Part model, mm, in its own coordinate system. Coordinates: 2 decimals unless noted, no trailing zeros. Loops run counter-clockwise (first coordinate to the right, second up) from the corner with the lowest first, then second, coordinate; pieces in that order, holes last. Notation, with made-up numbers: M -32,34 L 20,34 A25 ccw 20,61 Z; hole C 18.5,86 d10. An arc over 180 degrees is marked long. Use a Markdown table: item, result. Add a question column.
1) Band-saw the part on C-C (x = 5). List the corners of the cut face in (y, z).
2) Band-saw the part on A-A (x = 6). List the corners of the cut face in (y, z).
3) Pull direction Z, two halves, no side cores. Call faces 1 (the flat face through (5, 0.463, 1)), 2 (the flat face through (5, 5, 0)), 3 (the flat face through (5, 5, 2.5)): released by +Z, released by -Z, zero draft, split by the parting line, or undercut.
4) Band-saw the part on B-B (y = 1.75). List the corners of the cut face in (x, z).
5) Wall check: probe 1 along X at (y, z) = (8, 1.05); probe 2 along Z at (x, y) = (6.25, 6.25); probe 3 along Y at (x, z) = (2, 1.45). Give the ranges that are in metal, low to high. Write a range as from..to.
from build123d import *

# Parameters (mm, degrees)
CROQUIS1_W              = 9.859
CROQUIS1_H              = 2.5
CROQUIS1_W_2            = 0.636
CROQUIS1_H_2            = 0.636
SALIENTE_EXTRUIR2_DEPTH = 9.6
CHAFL_N2_SIZE           = 0.5
CHAFL_N3_SIZE           = 0.5
CROQUIS2_W              = 1.000954756
CROQUIS2_H              = 0.463176593
CORTAR_EXTRUIR1_DEPTH   = 10.859


with BuildPart() as part:
    # Croquis1 → Saliente-Extruir2 (new body)
    with BuildSketch(Plane(origin=(0, 0, 0), x_dir=(1, 0, 0), z_dir=(0, 1, 0))):
        with Locations((4.9295, -1.25)):
            Rectangle(CROQUIS1_W, CROQUIS1_H)
        with Locations((1.118, -1.25)):
            Rectangle(CROQUIS1_W_2, CROQUIS1_H_2, mode=Mode.SUBTRACT)
        with Locations((3.659, -1.25)):
            Rectangle(CROQUIS1_W_2, CROQUIS1_H_2, mode=Mode.SUBTRACT)
        with Locations((8.741, -1.25)):
            Rectangle(CROQUIS1_W_2, CROQUIS1_H_2, mode=Mode.SUBTRACT)
        with Locations((6.2, -1.25)):
            Rectangle(CROQUIS1_W_2, CROQUIS1_H_2, mode=Mode.SUBTRACT)
    extrude(amount=SALIENTE_EXTRUIR2_DEPTH)

    # Chaflán2
    chafl_n2_edges = [part.edges().sort_by_distance(p)[0] for p in [
        (0.8, 9.6, 1.25),
        (1.118, 9.6, 1.568),
        (1.436, 9.6, 1.25),
        (1.118, 9.6, 0.932),
    ]]
    chamfer(chafl_n2_edges, length=CHAFL_N2_SIZE)

    # Chaflán3
    chafl_n3_edges = [part.edges().sort_by_distance(p)[0] for p in [
        (3.659, 9.6, 0.932),
        (3.341, 9.6, 1.25),
        (3.659, 9.6, 1.568),
        (3.977, 9.6, 1.25),
        (8.741, 9.6, 0.932),
        (8.423, 9.6, 1.25),
        (8.741, 9.6, 1.568),
        (9.059, 9.6, 1.25),
        (6.2, 9.6, 0.932),
        (5.882, 9.6, 1.25),
        (6.2, 9.6, 1.568),
        (6.518, 9.6, 1.25),
    ]]
    chamfer(chafl_n3_edges, length=CHAFL_N3_SIZE)

    # Croquis2 → Cortar-Extruir1 (cut, through all)
    with BuildSketch(Plane.ZY):
        with Locations((1.236111308, 0.231588297)):
            Rectangle(CROQUIS2_W, CROQUIS2_H)
    extrude(amount=-CORTAR_EXTRUIR1_DEPTH, mode=Mode.SUBTRACT)


solid = part.part
Entries:
| question | item | result |
|---|---|---|
| 1 | outline | M 0,0 L 9.6,0 L 9.6,2.5 L 0,2.5 L 0,1.74 L 0.46,1.74 L 0.46,0.74 L 0,0.74 Z |
| 2 | outline | M 0,0 L 9.6,0 L 9.6,0.43 L 9.1,0.93 L 0.46,0.93 L 0.46,0.74 L 0,0.74 Z; M 0,1.74 L 0.46,1.74 L 0.46,1.57 L 9.1,1.57 L 9.6,2.07 L 9.6,2.5 L 0,2.5 Z |
| 3 | face 1 | undercut |
| 3 | face 2 | released by -Z |
| 3 | face 3 | released by +Z |
| 4 | outline | M 0,0 L 9.86,0 L 9.86,2.5 L 0,2.5 Z; hole M 0.8,0.93 L 1.44,0.93 L 1.44,1.57 L 0.8,1.57 Z; hole M 3.34,0.93 L 3.98,0.93 L 3.98,1.57 L 3.34,1.57 Z; hole M 5.88,0.93 L 6.52,0.93 L 6.52,1.57 L 5.88,1.57 Z; hole M 8.42,0.93 L 9.06,0.93 L 9.06,1.57 L 8.42,1.57 Z |
| 5 | probe 1 | 0..0.8, 1.44..3.34, 3.98..5.88, 6.52..8.42, 9.06..9.86 |
| 5 | probe 2 | 0..0.93, 1.57..2.5 |
| 5 | probe 3 | 0.46..9.6 |
